Work out the finished part from the listing and answer in its coordinate system (mm). Face numbers are marked on the shaded views. A direction names the side the tool comes from. Coordinates: 2 decimals unless noted, no trailing zeros. Write each loop counter-clockwise with the first axis right and the second up, starting at its lowest first coordinate (ties: lowest second). Pieces come first, ordered by that corner, then holes. Notation, with made-up numbers: (0.5, 65.5) - (31.5, 65.5) arc R27 ccw to (31.5, 93.5) - close; hole circle Ø5 at (-3, 72). An arc over 180 degrees is marked (long way). Answer as a JSON object with one key per item and string values. Group by question number.
from build123d import *

# Parameters (mm, degrees)
SKETCH1_W           = 53.5
SKETCH1_H           = 101.7
SKETCH1_R           = 1.5
BOSS_EXTRUDE1_DEPTH = 1.54
SKETCH2_W           = 2.5
SKETCH2_H           = 15.6
BOSS_EXTRUDE2_DEPTH = 8.25
SKETCH3_W           = 6
SKETCH3_H           = 6
BOSS_EXTRUDE3_DEPTH = 3.7
SKETCH5_R           = 1.785
BOSS_EXTRUDE5_DEPTH = 0.64
SKETCH4_W           = 45.5
SKETCH4_H           = 5
SKETCH4_W_2         = 2.5
SKETCH4_H_2         = 20
SKETCH4_W_3         = 5
SKETCH4_H_3         = 14.9
BOSS_EXTRUDE4_DEPTH = 2.5


with BuildPart() as part:
    # Sketch1 → Boss-Extrude1 (new body)
    with BuildSketch(Plane(origin=(0, 0, 0), x_dir=(1, 0, 0), z_dir=(0, 1, 0))):
        Rectangle(SKETCH1_W, SKETCH1_H)
        with Locations(Location((24.125, -39.35, 0), (0, 0, 270))):
            Circle(SKETCH1_R, mode=Mode.SUBTRACT)
        with Locations(Location((-24.125, -45.7, 0), (0, 0, 270))):
            Circle(SKETCH1_R, mode=Mode.SUBTRACT)
        with Locations(Location((24.125, 35.65, 0), (0, 0, 270))):
            Circle(SKETCH1_R, mode=Mode.SUBTRACT)
        with Locations(Location((-24.125, 35.65, 0), (0, 0, 270))):
            Circle(SKETCH1_R, mode=Mode.SUBTRACT)
    extrude(amount=BOSS_EXTRUDE1_DEPTH)

    # Sketch2 → Boss-Extrude2 (add)
    with BuildSketch(Plane(origin=(0, 1.54, 0), x_dir=(1, 0, 0), z_dir=(0, 1, 0))):
        with Locations((11.8, 11.35)):
            Rectangle(SKETCH2_W, SKETCH2_H)
        with Locations((-11.15, 11.35)):
            Rectangle(SKETCH2_W, SKETCH2_H)
    extrude(amount=BOSS_EXTRUDE2_DEPTH)

    # Sketch3 → Boss-Extrude3 (add)
    with BuildSketch(Plane(origin=(0, 1.54, 0), x_dir=(1, 0, 0), z_dir=(0, 1, 0))):
        with Locations((22.25, 45.15)):
            Rectangle(SKETCH3_W, SKETCH3_H)
    extrude(amount=BOSS_EXTRUDE3_DEPTH)

    # Sketch5 → Boss-Extrude5 (add)
    with BuildSketch(Plane(origin=(0, 5.24, 0), x_dir=(1, 0, 0), z_dir=(0, 1, 0))):
        with Locations(Location((22.25, 45.15, 0), (0, 0, 90))):
            Circle(SKETCH5_R)
    extrude(amount=BOSS_EXTRUDE5_DEPTH)

    # Sketch4 → Boss-Extrude4 (add)
    with BuildSketch(Plane.XZ):
        with Locations((2.86, 44.35)):
            Rectangle(SKETCH4_W, SKETCH4_H)
        with Locations((24.36, 25.85)):
            Rectangle(SKETCH4_W_2, SKETCH4_H_2)
        with Locations((23.11, 3.1)):
            Rectangle(SKETCH4_W_3, SKETCH4_H_2)
        with Locations((23.11, -18.4)):
            Rectangle(SKETCH4_W_3, SKETCH4_H_2)
        with Locations((-23.9, 31.95)):
            Rectangle(SKETCH4_W_2, SKETCH4_H_2)
        with Locations((-23.9, 9.2)):
            Rectangle(SKETCH4_W_2, SKETCH4_H_2)
        with Locations((-23.9, -11)):
            Rectangle(SKETCH4_W_2, SKETCH4_H_3)
    extrude(amount=BOSS_EXTRUDE4_DEPTH)


solid = part.part
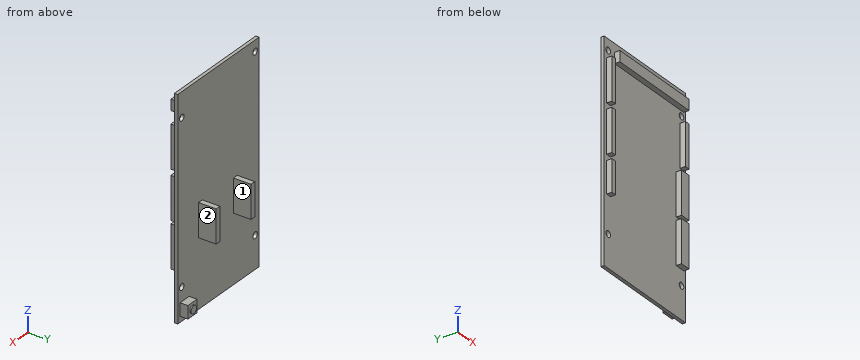
Q1. Section D-D on x = -2 is taken. Determine the outline of the cut face in (y, z), plus the area to 3 significant figures.
Q2. Consider L1, parallel to X at y = 0.9, z = -35.65 (3 decimals); L2, parallel to Z at x = 24.5, y = -2; L3, parallel to X at y = 1.2, z = 39.35 (3 decimals). Determine where each line is inside the solid, lowest interval first. Write a range as from..to.
Q3. Section C-C on z = -35.65 is taken. Determine the outline of the cut face in (x, y) (3 decimals).
Q4. Section A-A on y = 7.75 is taken. Determine the outline of the cut face in (x, z).
Q5. Section B-B on z = 45.7 is taken. Determine the outline of the cut face in (x, y) (3 decimals).
Q6. Flat-ended cylindrical pins translate along their axes: pin 1 Ø2 at (x, z) = (6.5, 36.5) entering from -Y; pin 2 Ø8 at (x, z) = (2, 26.5) entering from +Y; pin 3 Ø2 at (x, y) = (-12.5, 5.5) entering from -Z. Find the tip coordinate at first contact, or state that the pin passes through.
Q7. A tool of negligible diameter and unlimited length cuts with its end or side. For the marked faces 1 and 2, from which of +Z, -Z, +X, -X, +Y, -Y can it reach the whole face along a straight path? Write none if from no direction.
Numbers:
{
 "1": {"outline": "(-2.5, 41.85) - (0, 41.85) - (0, -50.85) - (1.54, -50.85) - (1.54, 50.85) - (0, 50.85) - (0, 46.85) - (-2.5, 46.85) - close", "area": "169 mm²"},
 "2": {"L1": "x = -26.75..-25.625, -22.625..22.625, 25.625..26.75", "L2": "z = -28.4..-8.4, -6.9..13.1, 15.85..35.85, 41.85..46.85", "L3": "x = -26.75..22.625, 25.625..26.75"},
 "3": {"outline": "(-26.75, 0) - (-25.625, 0) - (-25.625, 1.54) - (-26.75, 1.54) - close; (-22.625, 0) - (22.625, 0) - (22.625, 1.54) - (-22.625, 1.54) - close; (25.625, 0) - (26.75, 0) - (26.75, 1.54) - (25.625, 1.54) - close"},
 "4": {"outline": "(-12.4, -19.15) - (-9.9, -19.15) - (-9.9, -3.55) - (-12.4, -3.55) - close; (10.55, -19.15) - (13.05, -19.15) - (13.05, -3.55) - (10.55, -3.55) - close"},
 "5": {"outline": "(-26.75, 0) - (-25.625, 0) - (-25.625, 1.54) - (-26.75, 1.54) - close; (-22.625, 0) - (-19.89, 0) - (-19.89, -2.5) - (25.61, -2.5) - (25.61, 0) - (26.75, 0) - (26.75, 1.54) - (-22.625, 1.54) - close"},
 "6": {"pin 1": "stops at y = 0", "pin 2": "stops at y = 1.54", "pin 3": "stops at z = -19.15"},
 "7": {"face 1": "+Z, -Z, +Y", "face 2": "+Z, -Z, +X, +Y"}
}
